Geometry check sheet. Reference: the model listing, model coordinates, mm. Coordinates: 2 decimals unless noted, no trailing zeros. Loops run counter-clockwise (first coordinate to the right, second up) from the corner with the lowest first, then second, coordinate; pieces in that order, holes last. Notation, with made-up numbers: (77.25, 45) -> (135.25, 45) arc R24 cw to (135.25, 76) -> close; hole circle Ø8 at (27, 28.25). An arc over 180 degrees is marked (long way). Answer as a JSON object with one key per item and string values.
from build123d import *

# Parameters (mm, degrees)
EXTRUDE_1_DEPTH     = 4
SKETCH_2_R          = 1.5
CUT_EXTRUDE_1_DEPTH = 4
SKETCH_3_W          = 10
SKETCH_3_H          = 69.678883607
SKETCH_3_H_2        = 93.047687854
CUT_EXTRUDE_2_DEPTH = 4
CUT_EXTRUDE_3_DEPTH = 4
EXTRUDE_2_DEPTH     = 4


with BuildPart() as part:
    # 草图1 → 凸台-拉伸1 (new body)
    with BuildSketch(Plane(origin=(0, 0, 0), x_dir=(1, 0, 0), z_dir=(0, 1, 0))):
        Polygon((-67.5, -35), (-47.5, -15), (2.5, -15), (22.5, -35), (92.5, -35), (92.5, 15), (72.5, 35), (-117.5, 35), (-137.5, 15), (-137.5, -35), align=None)
    extrude(amount=EXTRUDE_1_DEPTH)

    # 草图2 → 切除-拉伸1 (cut)
    with BuildSketch(Plane(origin=(0, 4, 0), x_dir=(1, 0, 0), z_dir=(0, 1, 0))):
        with Locations(Location((-97.5, -15, 0), (0, 0, 270))):
            Circle(SKETCH_2_R)
        with Locations(Location((-97.5, 25, 0), (0, 0, 270))):
            Circle(SKETCH_2_R)
        with Locations(Location((52.5, 25, 0), (0, 0, 90))):
            Circle(SKETCH_2_R)
        with Locations(Location((52.5, -15, 0), (0, 0, 90))):
            Circle(SKETCH_2_R)
    extrude(amount=-CUT_EXTRUDE_1_DEPTH, mode=Mode.SUBTRACT)

    # 草图3 → 切除-拉伸2 (cut)
    with BuildSketch(Plane(origin=(0, 4, 0), x_dir=(1, 0, 0), z_dir=(0, 1, 0))):
        with Locations((-132.5, -0.160558196)):
            Rectangle(SKETCH_3_W, SKETCH_3_H)
        with Locations((87.5, 11.523843927)):
            Rectangle(SKETCH_3_W, SKETCH_3_H_2)
    extrude(amount=-CUT_EXTRUDE_2_DEPTH, mode=Mode.SUBTRACT)

    # 草图4 → 切除-拉伸3 (cut)
    with BuildSketch(Plane(origin=(0, 4, 0), x_dir=(1, 0, 0), z_dir=(0, 1, 0))):
        Polygon((-127.5, 12.5), (-92.197077218, 47.802922782), (-150.178982695, 47.802922782), align=None)
        Polygon((82.5, 12.5), (37.005283765, 57.994716235), (96.544114713, 56.205234398), align=None)
    extrude(amount=-CUT_EXTRUDE_3_DEPTH, mode=Mode.SUBTRACT)

    # 草图5 → 凸台-拉伸2 (add)
    with BuildSketch(Plane(origin=(0, 4, 0), x_dir=(1, 0, 0), z_dir=(0, 1, 0))):
        Polygon((-127.5, 12.5), (-132.5, 7.215634365), (-132.5, -35), (-127.5, -35), align=None)
        Polygon((82.5, -35), (82.5, 12.5), (87.5, 7.215634365), (87.5, -35), align=None)
    extrude(amount=-EXTRUDE_2_DEPTH)


solid = part.part
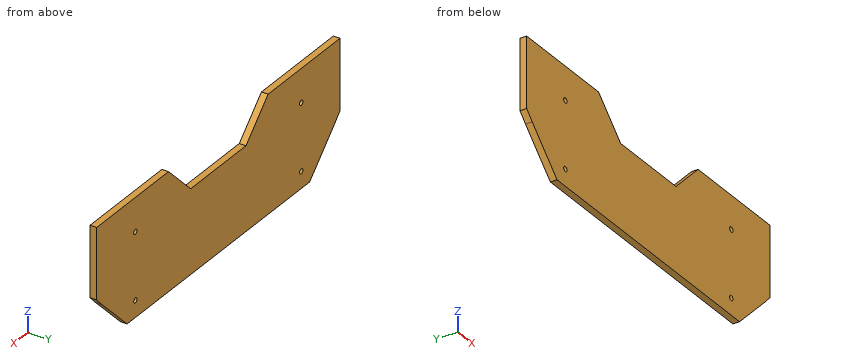
1. Section check D-D, the plane x = -116.5. Record the boundary of the cut face in (y, z).
Evaluation:
{"outline": "(0, -23.5) -> (4, -23.5) -> (4, 35) -> (0, 35) -> close"}
2. Section check B-B, the plane y = 0.65. Record the boundary of the cut face in (x, z).
Evaluation:
{"outline": "(-132.5, -7.22) -> (-127.5, -12.5) -> (-105, -35) -> (60, -35) -> (82.5, -12.5) -> (87.5, -7.22) -> (87.5, 35) -> (22.5, 35) -> (2.5, 15) -> (-47.5, 15) -> (-67.5, 35) -> (-132.5, 35) -> close; hole circle Ø3 at (-97.5, -25); hole circle Ø3 at (-97.5, 15); hole circle Ø3 at (52.5, -25); hole circle Ø3 at (52.5, 15)"}
3. Thickness scan on probe 1 along Z at (x, y) = (52.5, 2.95); probe 2 along Z at (x, y) = (53, 3.6); probe 3 along X at (y, z) = (2.45, -25). Record the ranges inside material, lowest first. Write a range as from..to.
Evaluation:
{"probe 1": "z = -35..-26.5, -23.5..13.5, 16.5..35", "probe 2": "z = -35..-26.41, -23.59..13.59, 16.41..35", "probe 3": "x = -115..-99, -96..51, 54..70"}
4. Section check A-A, the plane z = 27.5. Record the boundary of the cut face in (x, y), then the cut area to 3 significant figures.
Evaluation:
{"outline": "(-132.5, 0) -> (-60, 0) -> (-60, 4) -> (-132.5, 4) -> close; (15, 0) -> (87.5, 0) -> (87.5, 4) -> (15, 4) -> close", "area": "580 mm^2"}
5. Section check C-C, the plane x = -61. Record the boundary of the cut face in (y, z), then the cut area to 3 significant figures.
Evaluation:
{"outline": "(0, -35) -> (4, -35) -> (4, 28.5) -> (0, 28.5) -> close", "area": "254 mm^2"}
6. Depth check by flat-ended pin: P1, Ø2, axis at x = -16.5, y = 3.5, coming from the +Z side; P2, Ø3.5, axis at x = -97.5, z = -25, coming from the +Y side. Enter the tip coordinate at first touch or a pass-through.
Evaluation:
{"P1": "stops at z = 15", "P2": "stops at y = 4"}
